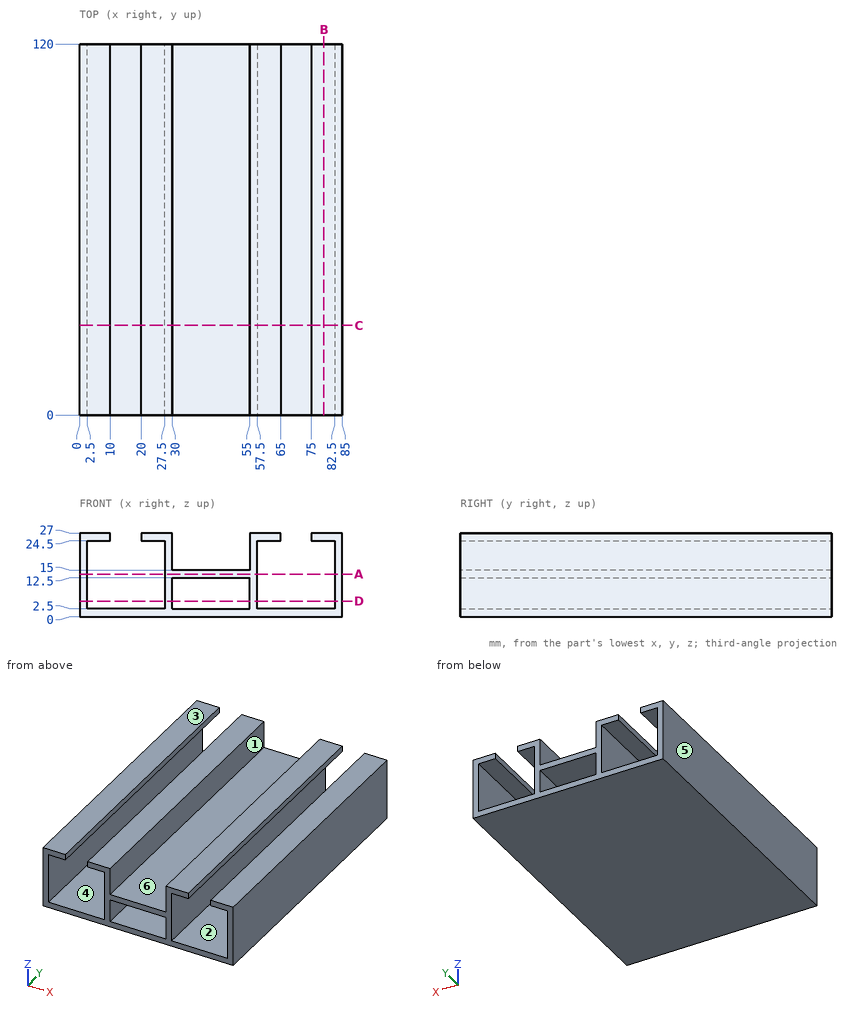
Geometry check sheet. Reference: drawing and pictorial views, mm from the part's lowest x, y, z. A direction names the side the tool comes from. Give positions to 0.01 mm unless a question says otherwise; leave off trailing zeros. Write each loop counter-clockwise with the first axis right and the second up, starting at its lowest first coordinate (ties: lowest second). Pieces come first, ordered by that corner, then holes. Notation, with made-up numbers: (86.5, -30) -> (100.5, -30) arc R24 ccw to (100.5, 6) -> close; hole circle Ø8 at (82.5, -10.75). An arc over 180 degrees is marked (long way). One line per question, with ' | ' between items.
Item 1: Sectioned sample at D-D, the plane z = 5. Record the boundary of the cut face in (x, y), plus the area to 3 significant figures.
Determined:
outline: (0, 0) -> (2.5, 0) -> (2.5, 120) -> (0, 120) -> close; (27.5, 0) -> (30, 0) -> (30, 120) -> (27.5, 120) -> close; (55, 0) -> (57.5, 0) -> (57.5, 120) -> (55, 120) -> close; (82.5, 0) -> (85, 0) -> (85, 120) -> (82.5, 120) -> close | area: 1,200 mm^2
Item 2: Sectioned sample at B-B, the plane x = 79. Record the boundary of the cut face in (y, z).
Determined:
outline: (0, 0) -> (120, 0) -> (120, 2.5) -> (0, 2.5) -> close; (0, 24.5) -> (120, 24.5) -> (120, 27) -> (0, 27) -> close
Item 3: Sectioned sample at C-C, the plane y = 29. Record the boundary of the cut face in (x, z).
Determined:
outline: (0, 0) -> (85, 0) -> (85, 27) -> (75, 27) -> (75, 24.5) -> (82.5, 24.5) -> (82.5, 2.5) -> (57.5, 2.5) -> (57.5, 24.5) -> (65, 24.5) -> (65, 27) -> (55, 27) -> (55, 15) -> (30, 15) -> (30, 27) -> (20, 27) -> (20, 24.5) -> (27.5, 24.5) -> (27.5, 2.5) -> (2.5, 2.5) -> (2.5, 24.5) -> (10, 24.5) -> (10, 27) -> (0, 27) -> close; hole (30, 2.5) -> (55, 2.5) -> (55, 12.5) -> (30, 12.5) -> close
Item 4: Scan lines: line 1 along X through (y, z) = (61, 20.5); line 2 along X through (y, z) = (58, 25); line 3 along Z through (x, y) = (51.5, 70). Record each from-to range of solid material in increasing order.
Determined:
line 1: 0 to 2.5, 27.5 to 30, 55 to 57.5, 82.5 to 85 | line 2: 0 to 10, 20 to 30, 55 to 65, 75 to 85 | line 3: 0 to 2.5, 12.5 to 15
Item 5: Depth check by flat-ended pin: pin 1 (7.5 mm diameter, centred on x = 70.5, y = 46, fed in from +Z). Enter the tip coordinate at first touch or a pass-through.
Determined:
pin 1: z = 2.5
Item 6: Sectioned sample at A-A, the plane z = 13.75. Record the boundary of the cut face in (x, y), plus the area to 3 significant figures.
Determined:
outline: (0, 0) -> (2.5, 0) -> (2.5, 120) -> (0, 120) -> close; (27.5, 0) -> (57.5, 0) -> (57.5, 120) -> (27.5, 120) -> close; (82.5, 0) -> (85, 0) -> (85, 120) -> (82.5, 120) -> close | area: 4,200 mm^2
Item 7: Draft check along Z on the marked faces 1, 2 and 3. Enter one of: released by +Z, released by -Z, zero draft, split by the parting line, or undercut.
Determined:
face 1: zero draft | face 2: undercut | face 3: released by +Z
Item 8: Access from +Z, -Z, +X, -X, +Y, -Y to the whole of each face (thin tool, end or side, straight path). Record for the marked faces 4, 5 and 6.
Determined:
face 4: +Y, -Y | face 5: +Z, -Z, -X, +Y, -Y | face 6: +Z, +Y, -Y
